Geometry: final body of the model. Coordinates: model frame, mm. A direction names the side the tool comes from. Coordinates: 2 decimals unless noted, no trailing zeros. Write item = value, one per line. Start each with the question number.
```python
from build123d import *

# Parameters (mm, degrees)
BOSS_EXTRUDE1_DEPTH = 70
SKETCH5_W           = 27.787302718
SKETCH5_H           = 26.03929452
CUT_EXTRUDE1_DEPTH  = 2.4


with BuildPart() as part:
    # Sketch4 → Boss-Extrude1 (new, symmetric)
    with BuildSketch(Plane.XY):
        with BuildLine():
            Line((3, -10), (8.25, -10))
            ThreePointArc((8.25, -10), (9.487436867, -9.487436867), (10, -8.25))
            Line((10, -8.25), (10, -3))
            ThreePointArc((10, -3), (9.853553391, -2.646446609), (9.5, -2.5))
            Line((9.5, -2.5), (8.424621202, -2.5))
            ThreePointArc((8.424621202, -2.5), (8.071067812, -2.646446609), (7.924621202, -3))
            Line((7.924621202, -3), (7.924621202, -5.25))
            ThreePointArc((7.924621202, -5.25), (7.615962919, -5.711939766), (7.071067812, -5.603553391))
            Line((7.071067812, -5.603553391), (4.478679656, -3.011165235))
            ThreePointArc((4.478679656, -3.011165235), (3.828361402, -2.037895189), (3.6, -0.889844892))
            Line((3.6, -0.889844892), (3.6, 0))
            Line((3.6, 0), (2.15, 0))
            ThreePointArc((2.15, 0), (1.52027958, -1.52027958), (0, -2.15))
            Line((0, -2.15), (0, -3.6))
            Line((0, -3.6), (0.889844892, -3.6))
            ThreePointArc((0.889844892, -3.6), (2.037895189, -3.828361402), (3.011165235, -4.478679656))
            Line((3.011165235, -4.478679656), (5.603553391, -7.071067812))
            ThreePointArc((5.603553391, -7.071067812), (5.711939766, -7.615962919), (5.25, -7.924621202))
            Line((5.25, -7.924621202), (3, -7.924621202))
            ThreePointArc((3, -7.924621202), (2.646446609, -8.071067812), (2.5, -8.424621202))
            Line((2.5, -8.424621202), (2.5, -9.5))
            ThreePointArc((2.5, -9.5), (2.646446609, -9.853553391), (3, -10))
        make_face()
    extrude(amount=BOSS_EXTRUDE1_DEPTH, both=True)

    # Mirror1: part across plane


with BuildPart() as part_1:
    add(part.part)
    add(part.part.mirror(Plane(origin=(0, 0, 0), x_dir=(0, 0, 1), z_dir=(1, 0, 0))))

    # Mirror2: part across plane


with BuildPart() as part_2:
    add(part_1.part)
    add(part_1.part.mirror(Plane.ZX))

    # Sketch5 → Cut-Extrude1 (cut)
    with BuildSketch(Plane.XY.offset(70)):
        with Locations((-0.060276145, -0.663037592)):
            Rectangle(SKETCH5_W, SKETCH5_H)
    extrude(amount=-CUT_EXTRUDE1_DEPTH, mode=Mode.SUBTRACT)


solid = part_2.part
```
Item 1: First-contact query: pin 1 (0.9 mm diameter, centred on x = 9, z = -34.5, fed in from -Y); pin 2 (1.4 mm diameter, centred on y = -0.5, z = -9, fed in from -X); pin 3 (0.9 mm diameter, centred on y = 9, z = -8.5, fed in from +X). Flat tips, straight axial feed; report the tip coordinate or a pass-through.
Item 2: Material intervals for probe 1 along Y at (x, z) = (3, 6); probe 2 along X at (y, z) = (7.5, 36); probe 3 along X at (y, z) = (0, -49), sorted ascending. Write a range as [from, to].
Item 3: Reachability of faces 1 (the flat face through (4.29, 5.76, -0.24)), 2 (the flat face through (-10, 6, 0)) from +Z, -Z, +X, -X, +Y, -Y: full face, straight path, thin tool, end or side. Return the list, or none.
Item 4: Draft query along X for faces 3 (the flat face through (-10, -6, 0)), 4 (the flat face through (-6, 10, 0)), 5 (the flat face through (-5.793, 4.326, -0.237)). Return one class per face: pulls with the +X half, pulls with the -X half, needs draft (parallel to the pull), parting line crosses it, or undercut.
Ans:
q1.pin_1 = -9.97
q1.pin_2 = -3.62
q1.pin_3 = 9.97
q2.probe_1 = [-10, -7.92], [-4.47, 4.47], [7.92, 10]
q2.probe_2 = [-10, -5.74], [5.74, 10]
q2.probe_3 = [-3.6, -2.15], [2.15, 3.6]
q3.face_1 = +Z, -Z
q3.face_2 = +Z, -Z, -X, +Y, -Y
q4.face_3 = pulls with the -X half
q4.face_4 = needs draft
q4.face_5 = undercut
